from build123d import *

# Parameters (mm, degrees)
F0_R           = 165.1
F1_DEPTH       = 25.4
F3_D           = 4.0386
F3_DEPTH       = 9.652
F3_TIP         = 1.213317848
F5_D           = 6.35
F5_CBORE_D     = 10.16
F5_CBORE_DEPTH = 12.7
F6_D           = 10.5
F7_D           = 2.2606
F7_DEPTH       = 10.16
F7_TIP         = 0.6791527577
F8_D           = 5.4102
F9_D           = 10.71626
F9_DEPTH       = 12.7
F9_TIP         = 3.2194893086


with BuildPart() as f1:
    # F0 (on Top) → F1 (new body)
    with BuildSketch(Plane.XY):
        Circle(F0_R)
    extrude(amount=-F1_DEPTH)

    # F3
    with Locations(Plane.XY):
        with Locations((-98.9867036526, 57.15), (-98.9867036526, -57.15), (0, -114.3), (98.9867036526, -57.15), (98.9867036526, 57.15), (0, 114.3)):
            Hole(F3_D / 2, depth=F3_DEPTH)
            with Locations((0, 0, -(F3_DEPTH + F3_TIP / 2))):  # 118° drill point
                Cone(0, F3_D / 2, F3_TIP, mode=Mode.SUBTRACT)

    # F5 (through all)
    with Locations(Plane(origin=(0, 0, -25.4), x_dir=(1, 0, 0), z_dir=(0, 0, -1))):
        with Locations((-134.9326057233, 55.8909152969), (-103.2729453923, 103.2729453923), (-55.8909152969, 134.9326057233), (0, 146.05), (55.8909152969, 134.9326057233), (103.2729453923, 103.2729453923), (134.9326057233, 55.8909152969), (146.05, 0), (134.9326057233, -55.8909152969), (103.2729453923, -103.2729453923), (55.8909152969, -134.9326057233), (0, -146.05), (-55.8909152969, -134.9326057233), (-103.2729453923, -103.2729453923), (-134.9326057233, -55.8909152969), (-146.05, 0)):
            CounterBoreHole(F5_D / 2, F5_CBORE_D / 2, F5_CBORE_DEPTH)

    # F6 (through all)
    with Locations(Plane(origin=(0, 0, -25.4), x_dir=(1, 0, 0), z_dir=(0, 0, -1))):
        with Locations((-127, 0)):
            Hole(F6_D / 2)

    # F7
    with Locations(Plane(origin=(0, 0, -25.4), x_dir=(1, 0, 0), z_dir=(0, 0, -1))):
        with Locations((140.462, -27.94)):
            Hole(F7_D / 2, depth=F7_DEPTH)
            with Locations((0, 0, -(F7_DEPTH + F7_TIP / 2))):  # 118° drill point
                Cone(0, F7_D / 2, F7_TIP, mode=Mode.SUBTRACT)

    # F8 (through all)
    with Locations(Plane(origin=(0, 0, -25.4), x_dir=(1, 0, 0), z_dir=(0, 0, -1))):
        with Locations((-58.58002, 101.4603)):
            Hole(F8_D / 2)

    # F9
    with Locations(Plane(origin=(0, 0, -25.4), x_dir=(1, 0, 0), z_dir=(0, 0, -1))):
        with Locations((63.5, -109.9852262806), (63.5, 109.9852262806)):
            Hole(F9_D / 2, depth=F9_DEPTH)
            with Locations((0, 0, -(F9_DEPTH + F9_TIP / 2))):  # 118° drill point
                Cone(0, F9_D / 2, F9_TIP, mode=Mode.SUBTRACT)


solid = f1.part
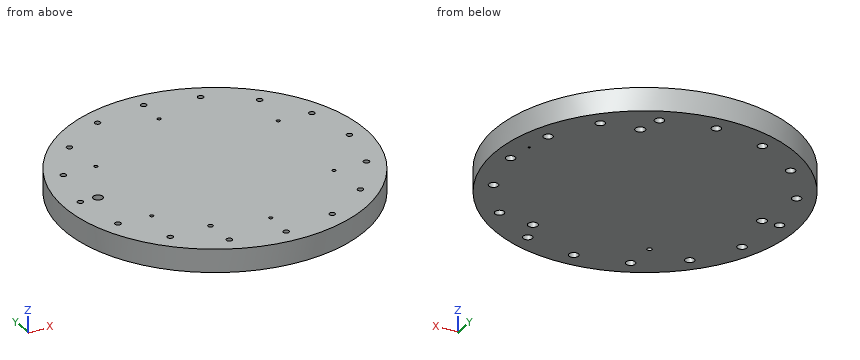
Geometry check sheet. Reference: the model listing, model coordinates, mm. Coordinates: 2 decimals unless noted, no trailing zeros. Order: outer loops, then holes, each group sorted by start corner. A loop starts at its lowest first (then second) coordinate and runs counter-clockwise, first axis right, second up. Notation, with made-up numbers: M 28,67.5 L 74,67.5 A9 ccw 74,83.5 Z; hole C 83.25,2.25 d11. An arc over 180 degrees is marked long. Use CSV: the item, a comma, the result in double quotes.
Item 1: Gauge pin test, flat ends, axial feed: pin 1 Ø8 at (x, y) = (-146.05, 0) entering from -Z; pin 2 Ø8 at (x, z) = (64, -10) entering from +Y; pin 3 Ø6 at (x, z) = (-58, -16) entering from -Y. Record the tip position at first contact, or that the pin passes through.
Returned:
pin 1,"stops at z = -12.7"
pin 2,"stops at y = 153.81"
pin 3,"stops at y = -155.67"
Item 2: Cross-section at A-A on z = -21.5. Give the number of separate pieces and of enclosed holes in the cut face, then the cut area to 3 significant figures.
Returned:
separate pieces,"1"
enclosed holes,"21"
area,"84,000 mm2"
Item 3: Cross-section at B-B on y = -74. Record the cut outline in (x, z), then the cut area to 3 significant figures.
Returned:
outline,"M -147.59,-25.4 L 147.59,-25.4 L 147.59,0 L -147.59,0 Z"
area,"7,500 mm2"
Item 4: Thickness scan on line 1 along Y through (x, z) = (0, -15.25); line 2 along Y through (x, z) = (0, -3.5) (3 decimals); line 3 along X through (y, z) = (-57.15, -7). Record the ranges inside material, lowest first.
Returned:
line 1,"y = -165.1 to -151.13, -140.97 to 140.97, 151.13 to 165.1"
line 2,"y = -165.1 to -149.225, -142.875 to -116.319, -112.281 to 112.281, 116.319 to 142.875, 149.225 to 165.1"
line 3,"x = -154.89 to -137.85, -132.02 to -101.01, -96.97 to 96.97, 101.01 to 132.02, 137.85 to 154.89"
Item 5: Cross-section at C-C on y = 91.5. Record the cut outline in (x, z).
Returned:
outline,"M -137.43,-25.4 L 137.43,-25.4 L 137.43,0 L -137.43,0 Z"
